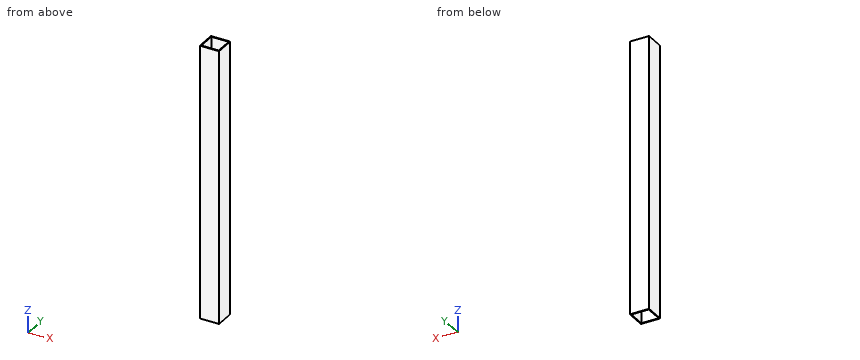
Autodesk Inventor part; units mm, degrees
ref_plane "YZ Plane" through (0, 0, 0) normal (1, 0, 0) x (0, 1, 0)
ref_plane "XZ Plane" through (0, 0, 0) normal (0, 1, 0) x (-1, 0, 0)
ref_plane "XY Plane" through (0, 0, 0) normal (0, 0, 1) x (1, 0, 0)
sketch "Sketch1" plane through (0, 0, 0) normal (0, 0, 1) x (1, 0, 0)
  line L0 (5.3443, -30.8421) -> (105.3443, -30.8421)
  line L1 (105.3443, -30.8421) -> (105.3443, 69.1579)
  line L2 (105.3443, 69.1579) -> (5.3443, 69.1579)
  line L3 (5.3443, 69.1579) -> (5.3443, -30.8421)
  line L4 (10.3443, 64.1579) -> (100.3443, 64.1579)
  line L5 (100.3443, 64.1579) -> (100.3443, -25.8421)
  line L6 (100.3443, -25.8421) -> (10.3443, -25.8421)
  line L7 (10.3443, -25.8421) -> (10.3443, 64.1579)
  point P0 (0, 0)
  dimension "d0" = 100
  dimension "d1" = 100
  dimension "d2" = 5
  dimension "d3" = 5
  dimension "d4" = 5
  dimension "d5" = 5
extrude "Extrusion1" add sketch "Sketch1" along normal blind 1420
properties part number "bluethingfortable"
The listing builds one solid part. Answer for the finished solid, in the listing's coordinates (mm). Give positions to 0.01 mm unless a question says otherwise; leave off trailing zeros. Order: outer loops, then holes, each group sorted by start corner. A loop starts at its lowest first (then second) coordinate and runs counter-clockwise, first axis right, second up. Notation, with made-up numbers: M 43.5,7 L 70.5,7 A28 cw 70.5,39 Z; hole C 40.5,-19.5 d10. An arc over 180 degrees is marked long. Put each result on its own line as item: value. Start each with the question number.
Item 1: The part is cut by section C-C, the plane x = 84. Determine the outline of the cut face in (y, z), and give its area (3 significant figures).
Item 2: The part is cut by section A-A, the plane y = 50.5. Determine the outline of the cut face in (x, z).
Item 3: Find the intervals of material crossed by line 1 along X through (y, z) = (-21.5, 654.5); line 2 along Y through (x, z) = (61, 99), in increasing order.
Item 4: The part is cut by section B-B, the plane z = 352.5. Determine the outline of the cut face in (x, y).
Answer key:
1. outline: M -30.84,0 L -25.84,0 L -25.84,1420 L -30.84,1420 Z; M 64.16,0 L 69.16,0 L 69.16,1420 L 64.16,1420 Z
1. area: 14,200 mm²
2. outline: M 5.34,0 L 10.34,0 L 10.34,1420 L 5.34,1420 Z; M 100.34,0 L 105.34,0 L 105.34,1420 L 100.34,1420 Z
3. line 1: x = 5.34 to 10.34, 100.34 to 105.34
3. line 2: y = -30.84 to -25.84, 64.16 to 69.16
4. outline: M 5.34,-30.84 L 105.34,-30.84 L 105.34,69.16 L 5.34,69.16 Z; hole M 10.34,-25.84 L 100.34,-25.84 L 100.34,64.16 L 10.34,64.16 Z
